Source: CAD feature listing. Evaluate the final solid. Frame: model axes, mm. Face numbers are marked on the shaded views. Coordinates: 2 decimals unless noted, no trailing zeros. Loops run counter-clockwise (first coordinate to the right, second up) from the corner with the lowest first, then second, coordinate; pieces in that order, holes last.
Autodesk Inventor part; units mm, degrees
ref_plane "YZ Plane" through (0, 0, 0) normal (1, 0, 0) x (0, 1, 0)
ref_plane "XZ Plane" through (0, 0, 0) normal (0, 1, 0) x (-1, 0, 0)
ref_plane "XY Plane" through (0, 0, 0) normal (0, 0, 1) x (1, 0, 0)
sketch "Sketch1" plane through (0, 0, 0) normal (0, 1, 0) x (-1, 0, 0)
  circle A0 centre (0, 0) radius 1.5875
  line L0 (3.175, 3.175) -> (-3.175, 3.175)
  line L1 (-3.175, 3.175) -> (-3.175, -15.24)
  line L2 (-3.175, -15.24) -> (3.175, -15.24)
  line L3 (3.175, -15.24) -> (3.175, 3.175)
  dimension "d0" = 3.175
  dimension "d1" = 3.175
  dimension "d2" = 3.175
  dimension "d3" = 3.175
  dimension "d4" = 15.24
extrude "Extrusion1" add sketch "Sketch1" along normal blind 1.5875
chamfer "Chamfer1" distance 1.27 angle 45 1 edges at (1.5875, 1.5875, 0)
sketch "Sketch2" plane through (0, 1.5875, 0) normal (0, 1, 0) x (1, 0, 0)
  line L0 (-3.175, 15.24) -> (-3.175, -3.175)
  line L1 (3.175, -3.175) -> (3.175, 15.24)
  circle A0 centre (0, 0) radius 2.8575
  circle A1 centre (9.2075, 14.4379) radius 1.5875
  circle A2 centre (9.2075, 14.4379) radius 3.175
  line L2 (9.2075, 17.6129) -> (3.175, 17.6129)
  line L3 (3.175, 0) -> (3.175, 15.875)
  line L4 (9.2075, 11.2629) -> (3.175, 11.2629)
  line L5 (-3.175, -3.175) -> (3.175, -3.175)
  line L6 (3.175, 15.24) -> (-3.175, 15.24)
  line L7 (3.175, 17.6129) -> (-3.175, 17.6129)
  line L8 (3.175, 15.24) -> (-3.175, 15.24)
  line L9 (-3.175, 17.6129) -> (-3.175, 15.24)
  line L10 (3.175, -3.175) -> (3.175, 15.24)
  line L11 (-3.175, 15.24) -> (3.175, 15.24)
  line L12 (3.175, 15.24) -> (3.175, 11.2629)
  dimension "d11" = 9.2075
  dimension "d12" = 14.4379
  dimension "d13" = 3.175
  dimension "d14" = 6.35
extrude "Extrusion3" add sketch "Sketch2" against normal up to surface (1.5875 mm away) contours L9 L7 L2 A2 L4 L1 L6 | A2
fillet "Fillet3" radius 3.175 4 edges at (3.175, 0.7937, -11.2629) (-3.175, 0.7937, -17.6129) (-3.175, 0.7937, 3.175) (3.175, 0.7937, 3.175)
chamfer "Chamfer3" distance 1.27 angle 45 1 edges at (7.62, 1.5875, -14.4379)
properties part number "limitSwitchHolder2Backplate" material "ABS Plastic"
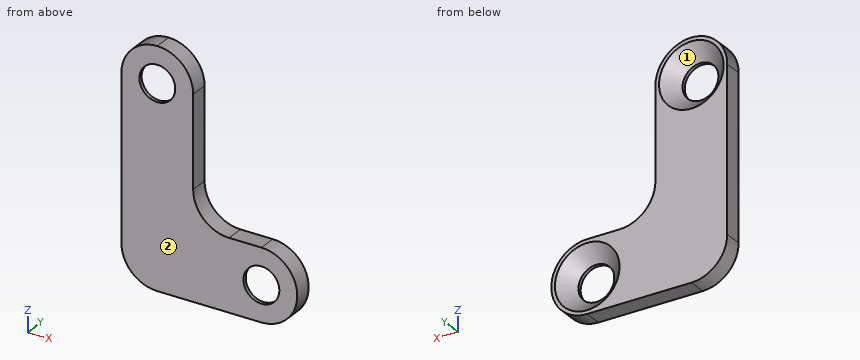
Q1. Section query A-A on y = 0.8. Count the separate pieces of the cut face and the enclosed holes in it, then the cut area to 3 significant figures.
Q2. Material intervals for line 1 along Z through (x, y) = (0, 0.25) (1 decimal); line 2 along Z through (x, y) = (6.25, 1.15); line 3 along X through (y, z) = (1.5, -16), sorted ascending.
Q3. Draft query along X for the marked faces 1 and 2. Return one class per face: released by +X, released by -X, zero draft, split by the parting line, or undercut.
Q4. First-contact query: pin 1 Ø5 at (x, z) = (9.21, -14.44) entering from -Y; pin 2 Ø0.5 at (y, z) = (1, -3) entering from +X (3 decimals); pin 3 Ø2.5 at (x, z) = (0, 0) entering from -Y. Flat tips, straight axial feed; report the tip coordinate or a pass-through.
Q5. Section query B-B on x = 3.5. Return the cut outline in (y, z), then the cut area to 3 significant figures.
Q6. Section query C-C on z = -4.5. Return the cut outline in (x, y) (1 decimal), then the cut area to 3 significant figures.
Resolved:
1. separate pieces: 1
1. enclosed holes: 2
1. area: 155 mm2
2. line 1: z = -17.6 to -1.6, 1.6 to 3.2
2. line 2: z = -17.61 to -11.26
2. line 3: x = -2.76 to 6.92, 11.5 to 11.97
3. face 1: undercut
3. face 2: zero draft
4. pin 1: stops at y = 0
4. pin 2: stops at x = 3.175
4. pin 3: passes through
5. outline: (0, -17.61) - (1.59, -17.61) - (1.59, -9.49) - (0, -9.49) - close
5. area: 12.9 mm2
6. outline: (-3.2, 0) - (3.2, 0) - (3.2, 1.6) - (-3.2, 1.6) - close
6. area: 10.1 mm2
